Verification items for the finished model (mm, model axes). Round coordinates to 2 decimals unless told otherwise and drop trailing zeros. Order: outer loops, then holes, each group sorted by start corner. A loop starts at its lowest first (then second) coordinate and runs counter-clockwise, first axis right, second up. Notation, with made-up numbers: (27, -27.75) -> (49, -27.75) arc R20 ccw to (49, -22.75) -> close; hole circle Ø6 at (-38.75, 86). An arc over 180 degrees is marked (long way). Answer in a Markdown table with one row per item. Add a question column.
```python
from build123d import *

# Parameters (mm, degrees)
SKETCH2_R          = 6.35
CUT_EXTRUDE1_DEPTH = 198.877910986
SKETCH3_R          = 12.7
CUT_EXTRUDE2_DEPTH = 198.877910986
SKETCH4_R          = 44.45
CUT_EXTRUDE3_DEPTH = 198.877910986


with BuildPart() as part:
    # Sketch1 → Revolve1 (revolve)
    with BuildSketch(Plane.XY, mode=Mode.PRIVATE) as revolve1_sk:
        with BuildLine():
            Line((0, 1.364957177), (0, -9.747542823))
            Line((0, -9.747542823), (120.65, -9.747542823))
            Line((120.65, -9.747542823), (120.65, -7.207542823))
            Line((120.65, -7.207542823), (127, -7.207542823))
            Line((127, -7.207542823), (127, -9.747542823))
            Line((127, -9.747542823), (139.7, -9.747542823))
            Line((139.7, -9.747542823), (139.7, -8.668042823))
            ThreePointArc((139.7, -8.668042823), (136.8425, -5.810542823), (139.7, -2.953042823))
            Line((139.7, -2.953042823), (139.7, 1.364957177))
            Line((139.7, 1.364957177), (137.16, 1.364957177))
            Line((137.16, 1.364957177), (137.16, 0.094957177))
            Line((137.16, 0.094957177), (130.81, 0.094957177))
            Line((130.81, 0.094957177), (130.81, 1.364957177))
            Line((130.81, 1.364957177), (0, 1.364957177))
        make_face()
    revolve(revolve1_sk.sketch.rotate(Axis((0, 12.263795045, 0), (0, -1, 0)), 90), axis=Axis((0, 12.263795045, 0), (0, -1, 0)))

    # Sketch2 → Cut-Extrude1 (cut, through all)
    with BuildSketch(Plane(origin=(0, 1.364957177, 0), x_dir=(1, 0, 0), z_dir=(0, 1, 0))):
        with Locations(Location((25.4, -50.8, 0), (0, 0, 270))):
            Circle(SKETCH2_R)
        with Locations(Location((-25.4, -50.8, 0), (0, 0, 270))):
            Circle(SKETCH2_R)
    extrude(amount=-CUT_EXTRUDE1_DEPTH, mode=Mode.SUBTRACT)

    # Sketch3 → Cut-Extrude2 (cut, through all)
    with BuildSketch(Plane(origin=(0, -9.747542823, 0), x_dir=(-1, 0, 0), z_dir=(0, -1, 0))):
        with Locations(Location((-25.4, 0, 0), (0, 0, 90))):
            Circle(SKETCH3_R)
        with Locations(Location((25.4, 0, 0), (0, 0, 90))):
            Circle(SKETCH3_R)
    extrude(amount=-CUT_EXTRUDE2_DEPTH, mode=Mode.SUBTRACT)

    # Sketch4 → Cut-Extrude3 (cut, through all)
    with BuildSketch(Plane(origin=(0, 1.364957177, 0), x_dir=(1, 0, 0), z_dir=(0, 1, 0))):
        with Locations(Location((0, 63.5, 0), (0, 0, 270))):
            Circle(SKETCH4_R)
    extrude(amount=-CUT_EXTRUDE3_DEPTH, mode=Mode.SUBTRACT)


solid = part.part
```
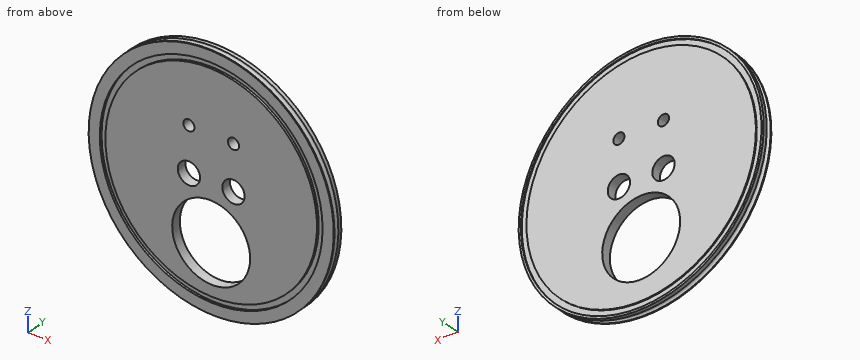
1) Cross-section at B-B, the plane z = 50.8. Give the number of separate pieces and of enclosed holes in the cut face, and give its area (3 significant figures).
2) Depth check by flat-ended pin: P1, Ø2, axis at x = 55, y = 0, coming from the -Z side; P2, Ø5, axis at y = -4.5, z = 105.5, coming from the +X side; P3, Ø2, axis at x = 45.5, y = -3, coming from the -Z side; P4, Ø16.5, axis at x = -25.4, z = 50.8, coming from the -Y side. Enter the tip coordinate at first touch or a pass-through.
3) Cross-section at C-C, the plane y = -5.5. Record the boundary of the cut face in (x, z).
4) Thickness scan on L1, parallel to X at y = -1.5, z = 0; L2, parallel to X at y = -0.5, z = 6.5; L3, parallel to Z at x = 23.5, y = -8.25. Record the ranges inside material, lowest first. Write a range as [from, to].
Results below:
| question | item | result |
|---|---|---|
| 1 | separate pieces | 3 |
| 1 | enclosed holes | 0 |
| 1 | area | 2,530 mm² |
| 2 | P1 | z = -128.84 |
| 2 | P2 | x = 93.79 |
| 2 | P3 | z = -132.42 |
| 2 | P4 | y = -9.75 |
| 3 | outline | circle Ø273.72 at (0, 0); hole circle Ø88.9 at (0, -63.5); hole circle Ø25.4 at (-25.4, 0); hole circle Ø12.7 at (-25.4, 50.8); hole circle Ø25.4 at (25.4, 0); hole circle Ø12.7 at (25.4, 50.8) |
| 4 | L1 | [-139.7, -38.1], [-12.7, 12.7], [38.1, 139.7] |
| 4 | L2 | [-139.55, -36.31], [-14.49, 14.49], [36.31, 139.55] |
| 4 | L3 | [-136.2, -124.81], [-118.34, -101.23], [-25.77, -12.56], [12.56, 44.74], [56.86, 118.34], [124.81, 136.2] |
